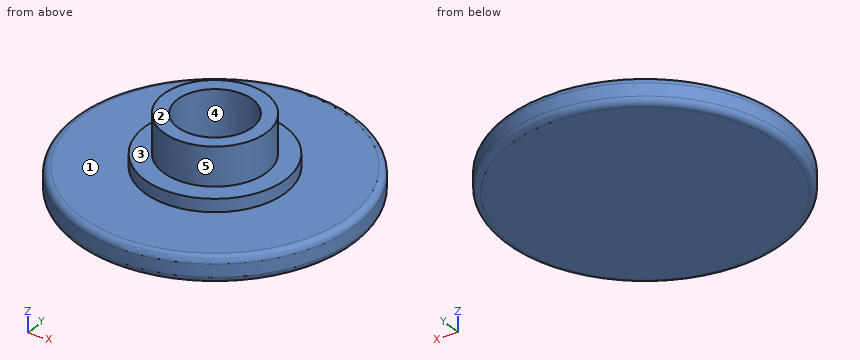
```python
from build123d import *

# Parameters (mm, degrees)
F0_R     = 10.95
F0_R_2   = 0.069
F3_DEPTH = 2
F1_R     = 5.5
F4_DEPTH = 3
F2_R     = 4.025
F5_DEPTH = 6
F6_R     = 0.5
F7_R     = 2.925
F8_DEPTH = 4


with BuildPart() as f3:
    # F0 (on Top) → F3 (new body)
    with BuildSketch(Plane.XY):
        Circle(F0_R)
        Circle(F0_R_2, mode=Mode.SUBTRACT)
    extrude(amount=F3_DEPTH)

    # F1 (on Top) → F4 (join)
    with BuildSketch(Plane.XY):
        Circle(F1_R)
    extrude(amount=F4_DEPTH)

    # F2 (on Top) → F5 (join)
    with BuildSketch(Plane.XY):
        Circle(F2_R)
    extrude(amount=F5_DEPTH)

    # F6
    f6_edges = [f3.edges().sort_by_distance(p)[0] for p in [
        (10.95, 0, 1),
        (-10.95, 0, 0),
        (-10.95, 0, 2),
    ]]
    fillet(f6_edges, radius=F6_R)

    # F7 (on face) → F8 (cut)
    with BuildSketch(Plane.XY.offset(6)):
        Circle(F7_R)
    extrude(amount=-F8_DEPTH, mode=Mode.SUBTRACT)


solid = f3.part
```
Model file for the job. Use its own axes, mm. Face numbers are marked on the shaded views. A direction names the side the tool comes from. Round coordinates to 2 decimals unless told otherwise and drop trailing zeros. Order: outer loops, then holes, each group sorted by start corner. A loop starts at its lowest first (then second) coordinate and runs counter-clockwise, first axis right, second up. Notation, with made-up numbers: (19, -17) -> (37, -17) arc R15 cw to (37, 1) -> close; hole circle Ø7 at (69.25, 10). An arc over 180 degrees is marked (long way). Use one line per item in the form item = value.
Item 1: Flat gauge pins, fed straight in: pin 1 Ø1.8 at (x, y) = (0.5, 0.5) entering from +Z; pin 2 Ø1 at (x, z) = (-7.5, 3) entering from +Y. Where does each tip first touch, or does it go through?
Returned:
pin_1 = 2
pin_2 = through
Item 2: Cut at A-A, the plane x = 0. Write the cut outline in (y, z) (3 decimals).
Returned:
outline = (-10.95, 0.5) arc R0.5 ccw to (-10.45, 0) -> (10.45, 0) arc R0.5 ccw to (10.95, 0.5) -> (10.95, 1.5) arc R0.5 ccw to (10.45, 2) -> (5.5, 2) -> (5.5, 3) -> (4.025, 3) -> (4.025, 6) -> (2.925, 6) -> (2.925, 2) -> (-2.925, 2) -> (-2.925, 6) -> (-4.025, 6) -> (-4.025, 3) -> (-5.5, 3) -> (-5.5, 2) -> (-10.45, 2) arc R0.5 ccw to (-10.95, 1.5) -> close
Item 3: Pull direction X, two halves, no side cores. Call the marked faces 3, 4 and 5: released by +X, released by -X, zero draft, split by the parting line, or undercut.
Returned:
face_3 = zero draft
face_4 = undercut
face_5 = split by the parting line
Item 4: Tool access for the marked faces 1 and 2: list every direction of +Z, -Z, +X, -X, +Y, -Y with a clear straight run to the whole face (end or side of a thin tool).
Returned:
face_1 = +Z
face_2 = +Z, +X, -X, +Y, -Y
Item 5: Drill centre lines: line 1 (Y direction, x = 0, z = 3.55) (3 decimals); line 2 (Z direction, x = 4, y = -5.25); line 3 (Z direction, x = -0.25, y = 4.75). Where is each one in solid material? Low to high.
Returned:
line_1 = -4.025 to -2.925, 2.925 to 4.025
line_2 = 0 to 2
line_3 = 0 to 3
Item 6: Cut at B-B, the plane z = 3.75. Write the cut outline in (x, y) (3 decimals).
Returned:
outline = circle Ø8.05 at (0, 0); hole circle Ø5.85 at (0, 0)
